Could you check a few things on this model? Use its own coordinates, in mm. A direction names the side the tool comes from. Coordinates: 2 decimals unless noted, no trailing zeros. Loops run counter-clockwise (first coordinate to the right, second up) from the corner with the lowest first, then second, coordinate; pieces in that order, holes last.
from build123d import *

# Parameters (mm, degrees)
F1_DEPTH = 15
F2_DEPTH = 7.5
F3_DEPTH = 15


with BuildPart() as f1:
    # F0 (on Front) → F1 (new body, symmetric)
    with BuildSketch(Plane.XZ):
        Polygon((40, 15), (0, 0), (40, 0), align=None)
        Polygon((30, 18.75), (10, 26.25), (10, 18.75), align=None)
        Polygon((0, 30), (0, 0), (40, 15), (30, 18.75), (10, 18.75), (10, 26.25), align=None)
    extrude(amount=F1_DEPTH, both=True)

    # F0 (on Front) → F2 (cut, symmetric)
    with BuildSketch(Plane.XZ):
        Polygon((30, 18.75), (10, 26.25), (10, 18.75), align=None)
    extrude(amount=F2_DEPTH, both=True, mode=Mode.SUBTRACT)

    # F0 (on Front) → F3 (cut, symmetric)
    with BuildSketch(Plane.XZ):
        Polygon((40, 15), (0, 0), (40, 0), align=None)
    extrude(amount=F3_DEPTH, both=True, mode=Mode.SUBTRACT)


solid = f1.part
(1) Which directions (+Z, -Z, +X, -X, +Y, -Y) give clear straight access to the entire face, cutting with the end or side of a thin tool? Please do faces 1 (the face through (15, -15, 15)), 2 (the face through (15, -7.5, 21)).
Answers:
face 1: +Z, -Z, +X, -X, -Y
face 2: +Z, +X
(2) Imagine slicing it at C-C, the plane z = 15.75. Write out the boundary of the cut face in (x, y), and give its area (3 significant figures).
Answers:
outline: (0, -15) - (38, -15) - (38, 15) - (0, 15) - close
area: 1,140 mm2
(3) For pin 1 (16.5 mm diameter, centred on x = 16.5, y = -2.5, fed in from +Z); pin 2 (4 mm diameter, centred on y = -0.5, z = 21, fed in from +X); pin 3 (4 mm diameter, centred on x = 19.5, y = -8.5, fed in from +Z), each with a flat end and sliding along its axis, tell me the tip position at first contact or that it passes through.
Answers:
pin 1: stops at z = 26.91
pin 2: stops at x = 10
pin 3: stops at z = 23.44
(4) Imagine slicing it at D-D, the plane x = 15.5. Write out the boundary of the cut face in (y, z).
Answers:
outline: (-15, 5.81) - (15, 5.81) - (15, 24.19) - (7.5, 24.19) - (7.5, 18.75) - (-7.5, 18.75) - (-7.5, 24.19) - (-15, 24.19) - close
(5) I need wall thicknesses on probe 1 along Y at (x, z) = (10.5, 24.75); probe 2 along X at (y, z) = (-5.5, 22); probe 3 along Z at (x, y) = (24, 9.5). Which ranges of each line are inside material? Lowest first, please.
Answers:
probe 1: y = -15 to -7.5, 7.5 to 15
probe 2: x = 0 to 10
probe 3: z = 9 to 21
(6) Imagine slicing it at A-A, the plane y = -6.25. Write out the boundary of the cut face in (x, z).
Answers:
outline: (0, 0) - (40, 15) - (30, 18.75) - (10, 18.75) - (10, 26.25) - (0, 30) - close
(7) We'd pull the mould along Y, two halves only. Please class faces 3 (the face through (10, 0, 23)), 4 (the face through (0, 0, 15)), 5 (the face through (15, 15, 15)): +Y half, -Y half, draft (parallel to the pull), parting line (faces both ways), or undercut.
Answers:
face 3: undercut
face 4: draft
face 5: +Y half
(8) Imagine slicing it at B-B, the plane x = 11. Write out the boundary of the cut face in (y, z) (3 decimals), and give its area (3 significant figures).
Answers:
outline: (-15, 4.125) - (15, 4.125) - (15, 25.875) - (7.5, 25.875) - (7.5, 18.75) - (-7.5, 18.75) - (-7.5, 25.875) - (-15, 25.875) - close
area: 546 mm2
